The model under review builds one solid part; all positions refer to its coordinate system, in mm. Face numbers are marked on the shaded views. A direction names the side the tool comes from. Round coordinates to 2 decimals unless told otherwise and drop trailing zeros. Order: outer loops, then holes, each group sorted by start corner. A loop starts at its lowest first (then second) coordinate and runs counter-clockwise, first axis right, second up.
1) Machinability: for the marked faces 1, 2 and 3, which of the approach directions +Z, -Z, +X, -X, +Y, -Y give a long, thin tool a straight path to every point of the face, cutting with its end or side? Answer none if there is none.
2) Mouldability with a two-part tool opening along X and no side actions: class the marked faces 4, 5, 6 and 7 as pulls with the +X half, pulls with the -X half, needs draft (parallel to the pull), parting line crosses it, or undercut.
3) Clearance check with flat-ended pins moving along their axes: P1, Ø10, axis at x = 13, y = 12, coming from the +Z side; P2, Ø20.5, axis at x = 16, z = 23.5, coming from the +Y side; P3, Ø2, axis at x = 64.5, y = 8.5, coming from the -Z side. State where each tip first meets the part, or that it passes through.
4) To check wall thickness, follow L1, parallel to X at y = 18.5, z = 20.5; L2, parallel to Z at x = 158, y = 12.75; L3, parallel to Z at x = 23, y = 16.25. State the ranges of each line that lie inside material, in increasing order.
5) Consider section C-C (y = 2.5). Give the boundary of the cut face in (x, z), then the cut area to 3 significant figures.
from build123d import *

# Parameters (mm, degrees)
F0_W      = 206.3
F0_H      = 52
F1_DEPTH  = 2.5
F2_SIZE   = 2.49999
F3_W      = 200.3
F3_H      = 46
F4_DEPTH  = 20
F5_W      = 196.3
F5_H      = 42
F6_DEPTH  = 25
F7_SIZE   = 1.5
F8_DEPTH  = 47
F9_W      = 43.8446728513
F9_H      = 40.8840479795
F10_DEPTH = 20.5


# Not quite as in the source:
# - a fillet or chamfer is up to 0.001 mm smaller than in the source, because OpenCascade refuses the exact size


with BuildPart() as f1:
    # F0 (on Front) → F1 (new body)
    with BuildSketch(Plane.XZ):
        with Locations((81.9657886937, 18.1555162981)):
            Rectangle(F0_W, F0_H)
    extrude(amount=F1_DEPTH)

    # F2 (size 2.5 in the source; OpenCascade refuses exactly that, so slightly less here)
    f2_edges = [f1.edges().sort_by_distance(p)[0] for p in [
        (81.965789, -2.5, 44.155516),
        (81.965789, -2.5, -7.844484),
        (185.115789, -2.5, 18.155516),
        (-21.184211, -2.5, 18.155516),
    ]]
    chamfer(f2_edges, length=F2_SIZE)

    # F3 (on face) → F4 (join)
    with BuildSketch(Plane(origin=(0, 0, 0), x_dir=(-1, 0, 0), z_dir=(0, 1, 0))):
        with Locations((-82.0777288884, 18.0567920078)):
            Rectangle(F3_W, F3_H)
    extrude(amount=F4_DEPTH)

    # F5 (on face) → F6 (cut)
    with BuildSketch(Plane(origin=(0, 20, 0), x_dir=(-1, 0, 0), z_dir=(0, 1, 0))):
        with Locations((-82.0056978608, 17.9472315861)):
            Rectangle(F5_W, F5_H)
    extrude(amount=-F6_DEPTH, mode=Mode.SUBTRACT)

    # F7
    f7_edges = [f1.edges().sort_by_distance(p)[0] for p in [
        (182.227729, 10, 41.056792),
        (182.227729, 10, -4.943208),
        (-18.072271, 10, 41.056792),
        (-18.072271, 10, -4.943208),
    ]]
    chamfer(f7_edges, length=F7_SIZE)

    # F8 (add): a face of the model
    f8_faces = [f1.faces().sort_by_distance(p)[0] for p in [
        (-16.1443021392, 8.75, 17.9472315861),
    ]]
    extrude(f8_faces, amount=F8_DEPTH)

    # F9 (on face) → F10 (cut)
    with BuildSketch(Plane(origin=(0, 20, 0), x_dir=(-1, 0, 0), z_dir=(0, 1, 0))):
        with Locations((-6.3970577903, 18.1101224152)):
            Rectangle(F9_W, F9_H)
    extrude(amount=-F10_DEPTH, mode=Mode.SUBTRACT)


solid = f1.part
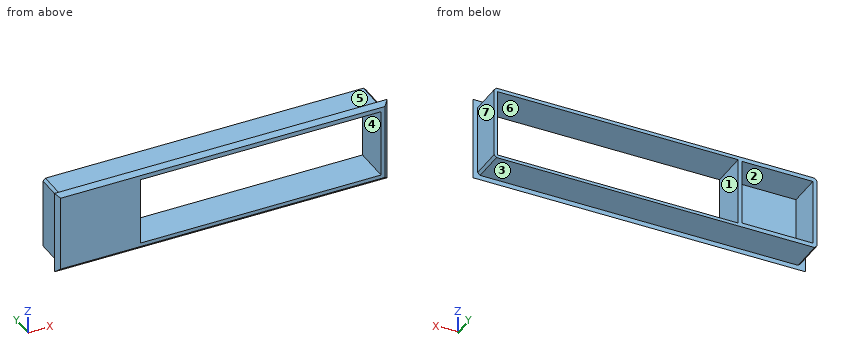
Answer below:
1. face 1: +Y, -Y
1. face 2: +Y
1. face 3: -Z, +X, -X, +Y
2. face 4: undercut
2. face 5: needs draft
2. face 6: undercut
2. face 7: pulls with the +X half
3. P1: stops at z = 41.06
3. P2: stops at y = -0.5
3. P3: stops at z = -4.94
4. L1: x = -18.07 to -15.53, 28.32 to 30.86, 180.16 to 182.23
4. L2: z = -4.94 to -3.05, 38.95 to 41.06
4. L3: z = -4.94 to -2.33, 38.55 to 41.06
5. outline: (-18.07, -3.44) - (-16.57, -4.94) - (180.73, -4.94) - (182.23, -3.44) - (182.23, 39.56) - (180.73, 41.06) - (-16.57, 41.06) - (-18.07, 39.56) - close; hole (-15.53, -2.33) - (28.32, -2.33) - (28.32, 38.55) - (-15.53, 38.55) - close; hole (30.86, -3.05) - (180.16, -3.05) - (180.16, 38.95) - (30.86, 38.95) - close
5. area: 1,150 mm2
